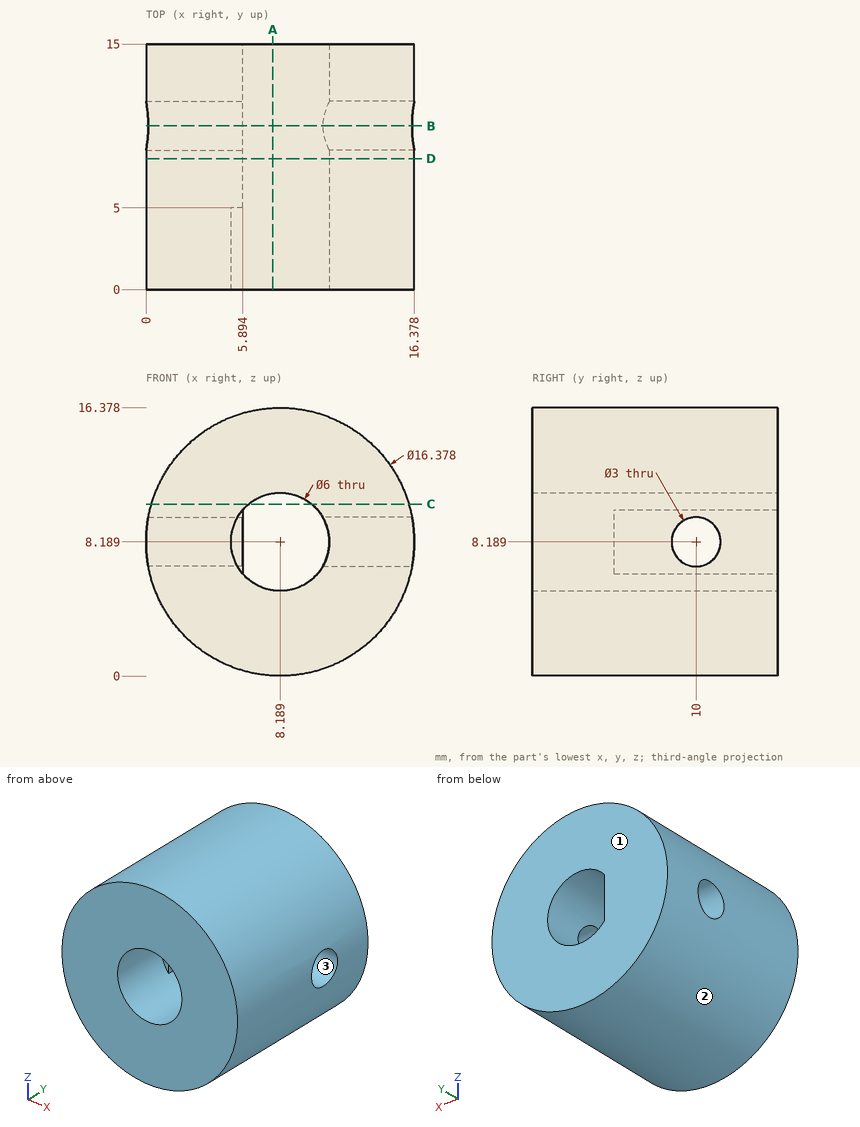
Source: three-view drawing plus pictorial views. Frame: mm from the lowest corner of the part. Round coordinates to 2 decimals unless told otherwise and drop trailing zeros. Loops run counter-clockwise (first coordinate to the right, second up) from the corner with the lowest first, then second, coordinate; pieces in that order, holes last. Notation, with made-up numbers: (-20, 36) - (-11, 36) arc R26 cw to (-11, 70) - close; hole circle Ø10 at (-2, 62). An arc over 180 degrees is marked (long way). Write item = value, one per line. Start each with the question number.
Item 1: First-contact query: pin 1 Ø1 at (x, y) = (3, 2) entering from -Z; pin 2 Ø4 at (y, z) = (7, 14.5) entering from -X; pin 3 Ø1 at (x, y) = (9, 10) entering from +Z; pin 4 Ø2.5 at (y, z) = (10, 8.19) entering from +X. Flat tips, straight axial feed; report the tip coordinate or a pass-through.
Item 2: Section query D-D on y = 8. Output: boundary loops of the cut face in (x, z).
Item 3: Material intervals for line 1 (Z direction, x = 8, y = 3.75) (3 decimals); line 2 (Z direction, x = 10.5, y = 10) (1 decimal); line 3 (X direction, y = 3, z = 7.5), sorted ascending.
Item 4: Mould query, pull axis Z, two halves, no side actions, for the marked faces 1, 2 and 3. Classes: released by +Z, released by -Z, zero draft, split by the parting line, or undercut.
Item 5: Section query A-A on x = 7.75. Output: boundary loops of the cut face in (y, z), plus the area to 3 significant figures.
Item 6: Section query C-C on z = 10.5. Output: boundary loops of the cut face in (x, y) (3 decimals).
Item 7: Section query B-B on y = 10. Output: boundary loops of the cut face in (x, z), plus the area to 3 significant figures.
Results list:
q1.pin_1 = 1.48
q1.pin_2 = 1.23
q1.pin_3 = 16.37
q1.pin_4 = through
q2.outline = circle Ø16.38 at (8.19, 8.19); hole (5.89, 6.26) arc R3 ccw (long way) to (5.89, 10.12) - close
q3.line_1 = 0.002 to 5.195, 11.183 to 16.376
q3.line_2 = 0.3 to 6.3, 10.1 to 16
q3.line_3 = 0.03 to 5.27, 11.11 to 16.35
q4.face_1 = zero draft
q4.face_2 = split by the parting line
q4.face_3 = undercut
q5.outline = (0, 0.01) - (15, 0.01) - (15, 5.22) - (0, 5.22) - close; (0, 11.16) - (15, 11.16) - (15, 16.37) - (0, 16.37) - close
q5.area = 156 mm²
q6.outline = (0.333, 0) - (6.276, 0) - (6.276, 15) - (0.333, 15) - close; (10.102, 0) - (16.045, 0) - (16.045, 15) - (10.102, 15) - close
q7.outline = (0.14, 6.69) arc R8.19 ccw to (16.24, 6.69) - (10.79, 6.69) arc R3 cw to (5.89, 6.26) - (5.89, 6.69) - close; (0.14, 9.69) - (5.89, 9.69) - (5.89, 10.12) arc R3 cw to (10.79, 9.69) - (16.24, 9.69) arc R8.19 ccw to start
q7.area = 151 mm²
